Geometry check sheet. Reference: drawing and pictorial views, mm from the part's lowest x, y, z. A direction names the side the tool comes from. Give positions to 0.01 mm unless a question says otherwise; leave off trailing zeros. Write each loop counter-clockwise with the first axis right and the second up, starting at its lowest first coordinate (ties: lowest second). Pieces come first, ordered by that corner, then holes. Notation, with made-up numbers: M 2,-29 L 31,-29 A17 cw 31,-24 Z; hole C 66.25,30 d2. An arc over 180 degrees is marked long. Answer as a JSON object with one key per item and string values.
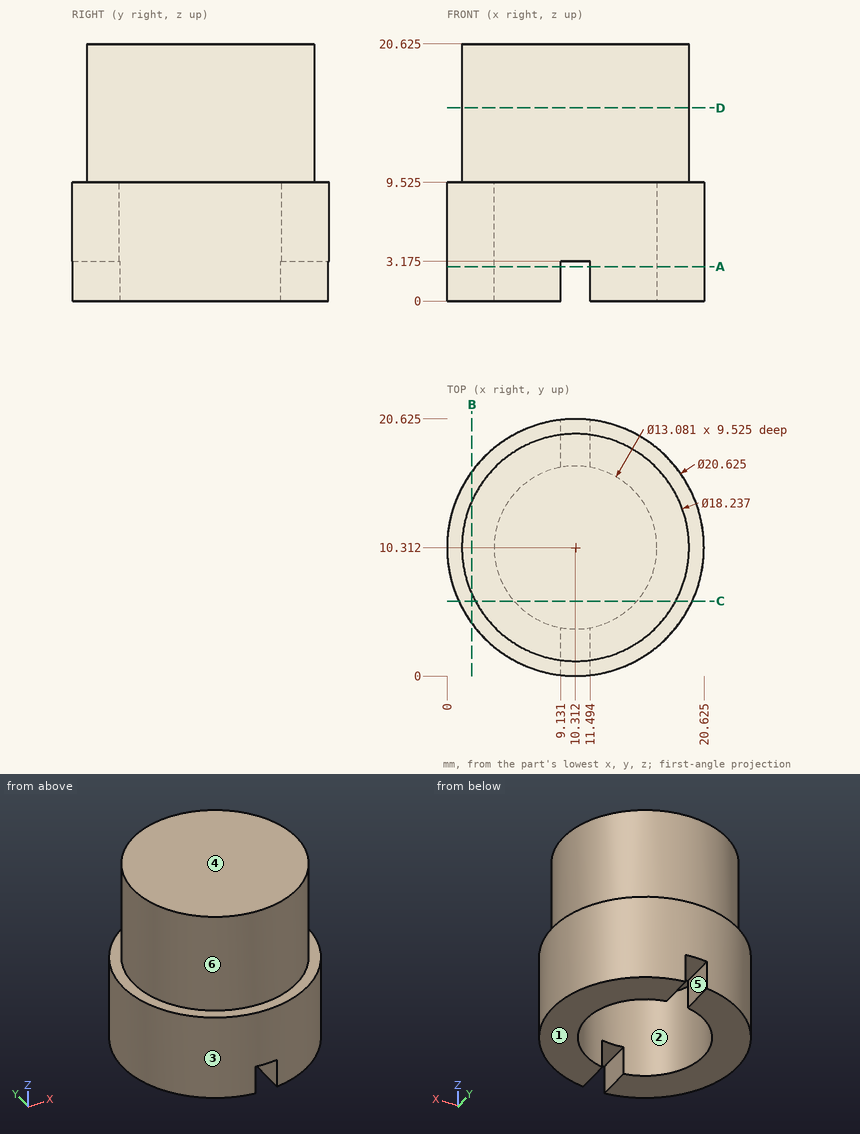
1) Access from +Z, -Z, +X, -X, +Y, -Y to the whole of each face (thin tool, end or side, straight path). Record for the marked faces 4, 5 and 6.
Completed:
{"face 4": "+Z, +X, -X, +Y, -Y", "face 5": "-Z, +Y, -Y", "face 6": "+Z"}
2) Thickness scan on L1, parallel to Y at x = 11.5, z = 6.75 (1 decimal); L2, parallel to Z at x = 8.75, y = 4.75 (1 decimal); L3, parallel to X at y = 9.5, z = 7.5. Record the ranges inside material, lowest first.
Completed:
{"L1": "y = 0.1 to 3.9, 16.7 to 20.6", "L2": "z = 9.5 to 20.6", "L3": "x = 0.03 to 3.82, 16.8 to 20.59"}
3) Release check for a two-part mould opening along Y. For the marked faces 1, 2 and 3 record: pulls with the +Y half, pulls with the -Y half, needs draft (parallel to the pull), parting line crosses it, or undercut.
Completed:
{"face 1": "needs draft", "face 2": "undercut", "face 3": "parting line crosses it"}
4) Go/stop test with flat-tipped pins: pin 1 (1.5 mm diameter, centred on y = 15, z = 13.5, fed in from -X); pin 2 (1.5 mm diameter, centred on y = 9.5, z = 4.5, fed in from +X) (1 decimal); pin 3 (4 mm diameter, centred on x = 11, y = 12.5, fed in from -Z) (1 decimal); pin 4 (0.7 mm diameter, centred on x = 10, y = 19, fed in from -Z) (1 decimal). Record where each tip stops, or that it passes through.
Completed:
{"pin 1": "stops at x = 2.09", "pin 2": "stops at x = 20.6", "pin 3": "stops at z = 9.5", "pin 4": "stops at z = 3.2"}
5) Section check C-C on y = 6. Record the boundary of the cut face in (x, z) (1 decimal), and give its area (3 significant figures).
Completed:
{"outline": "M 0.9,0 L 5.4,0 L 5.4,9.5 L 15.2,9.5 L 15.2,0 L 19.7,0 L 19.7,9.5 L 18.3,9.5 L 18.3,20.6 L 2.3,20.6 L 2.3,9.5 L 0.9,9.5 Z", "area": "263 mm2"}
6) Section check D-D on z = 15.5. Record the boundary of the cut face in (x, y), and give its area (3 significant figures).
Completed:
{"outline": "C 10.31,10.31 d18.24", "area": "261 mm2"}
7) Section check A-A on z = 2.75. Record the boundary of the cut face in (x, y) (1 decimal).
Completed:
{"outline": "M 9.1,0.1 L 9.1,3.9 A6.5 cw 9.1,16.7 L 9.1,20.6 A10.3 ccw Z; M 11.5,0.1 A10.3 ccw 11.5,20.6 L 11.5,16.7 A6.5 cw 11.5,3.9 Z"}
8) Section check B-B on x = 2. Record the boundary of the cut face in (y, z) (1 decimal).
Completed:
{"outline": "M 4.2,0 L 16.4,0 L 16.4,9.5 L 14.1,9.5 L 14.1,20.6 L 6.6,20.6 L 6.6,9.5 L 4.2,9.5 Z"}
